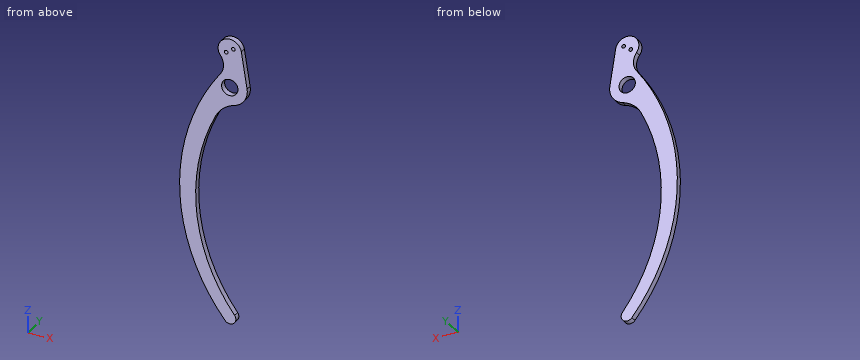
from build123d import *

# Parameters (mm, degrees)
F0_R     = 4.445
F0_R_2   = 1.016
F1_DEPTH = 3.175


with BuildPart() as f1:
    # F0 (on Front) → F1 (new body)
    with BuildSketch(Plane.XZ):
        with BuildLine():
            Line((9.40801, 1.488281), (6.272006, 21.312188))
            ThreePointArc((6.272006, 21.312188), (-2.482691, 26.164548), (-5.068596, 16.494842))
            ThreePointArc((-5.068596, 16.494842), (-3.37124, 11.428014), (-5.068596, 6.361186))
            ThreePointArc((-5.068596, 6.361186), (-27.200848, -61.795162), (-2.560215, -129.085307))
            ThreePointArc((-2.560215, -129.085307), (2.052999, -129.586194), (2.611765, -124.979632))
            ThreePointArc((2.611765, -124.979632), (-18.059382, -72.719897), (-7.62, -17.498565))
            ThreePointArc((-7.62, -17.498565), (-3.418112, -12.26682), (2.54, -9.180089))
            ThreePointArc((2.54, -9.180089), (8.008886, -5.155906), (9.40801, 1.488281))
        make_face()
        Circle(F0_R, mode=Mode.SUBTRACT)
        with Locations((-1.950606, 18.954171)):
            Circle(F0_R_2, mode=Mode.SUBTRACT)
        with Locations((1.950606, 21.685829)):
            Circle(F0_R_2, mode=Mode.SUBTRACT)
    extrude(amount=F1_DEPTH)


solid = f1.part
For this review, take the finished solid that the model builds, in its own axes (mm). Round coordinates to 2 decimals unless told otherwise and drop trailing zeros. Write each loop counter-clockwise with the first axis right and the second up, starting at its lowest first coordinate (ties: lowest second). Pieces come first, ordered by that corner, then holes. Notation, with made-up numbers: (-40, 6.5) - (12, 6.5) arc R16 cw to (12, 19.5) - close; hole circle Ø1 at (81.25, 62.5). An arc over 180 degrees is marked (long way). Write item = value, one per line. Start each with the question number.
1. Consider section D-D on z = -127. State the section outline as (x, y) points (3 decimals).
2. Consider section A-A on z = 0. State the section outline as (x, y) points (3 decimals).
3. Consider section C-C on y = -0.5. Give the number of separate pieces and of enclosed holes in the cut face, plus the area to 3 significant figures.
4. For pin 1 Ø1.5 at (x, y) = (-2, -1.5) entering from -Z; pin 2 Ø8 at (x, z) = (0, 0) entering from +Y, all flat-tipped, find the tip position at first contact; note any pin that passes through.
5. Wall thickness on L1, parallel to Z at x = -2.5, y = -2.1; L2, parallel to Z at x = -10, y = -1.85; L3, parallel to Z at x = -9.5, y = -2.6: over which ranges is each line inside the solid? List them lowest first.
6. Consider section B-B on x = -12. State the section outline as (y, z) points (3 decimals), plus the area to 3 significant figures.
Evaluation:
q1.outline = (-4.217, -3.175) - (3.302, -3.175) - (3.302, 0) - (-4.217, 0) - close
q2.outline = (-9.525, -3.175) - (-4.445, -3.175) - (-4.445, 0) - (-9.525, 0) - close; (4.445, -3.175) - (9.525, -3.175) - (9.525, 0) - (4.445, 0) - close
q3.separate_pieces = 1
q3.enclosed_holes = 3
q3.area = 1,540 mm2
q4.pin_1 = -130.06
q4.pin_2 = through
q5.L1 = -129.16 to -117.74, -11.57 to -3.68, 3.68 to 18.1, 19.81 to 26.16
q5.L2 = -118.79 to -103.74, -22.54 to -0.74
q5.L3 = -119.56 to -104.86, -21.42 to 0.04
q6.outline = (-3.175, -115.527) - (0, -115.527) - (0, -98.839) - (-3.175, -98.839) - close; (-3.175, -27.445) - (0, -27.445) - (0, -3.998) - (-3.175, -3.998) - close
q6.area = 127 mm2
